Build history of the part. All positions in model axes, mm. A direction names the side the tool comes from. Coordinates: 2 decimals unless noted, no trailing zeros. Order: outer loops, then holes, each group sorted by start corner. A loop starts at its lowest first (then second) coordinate and runs counter-clockwise, first axis right, second up. Notation, with made-up numbers: (73.25, 74.25) - (129.25, 74.25) arc R25 cw to (129.25, 109.25) - close; hole circle Ø11 at (56.25, -35.75). An arc over 180 degrees is marked (long way). Return JSON: item names as keys, results as strings.
from build123d import *

# Parameters (mm, degrees)
SKETCH_1_W            = 62
SKETCH_1_H            = 98
EXTRUDE_1_DEPTH       = 8
CHAMFER_1_SIZE        = 1
HOLE_WIZARD_M4_1_D    = 4.8
CUT_EXTRUDE_1_DEPTH   = 3.3
MIRROR_2_COPY_1_D     = 4.8
MIRROR_2_COPY_2_DEPTH = 3.3


with BuildPart() as part:
    # ｽｹｯﾁ1 → ﾎﾞｽ - 押し出し1 (new body)
    with BuildSketch(Plane.XY):
        Rectangle(SKETCH_1_W, SKETCH_1_H)
    extrude(amount=EXTRUDE_1_DEPTH)

    # 面取り1
    chamfer_1_edges = [part.edges().sort_by_distance(p)[0] for p in [
        (0, -49, 0),
        (-31, 0, 0),
        (0, 49, 0),
        (31, 0, 0),
        (31, -49, 4),
        (-31, -49, 4),
        (-31, 49, 4),
        (31, 49, 4),
    ]]
    chamfer(chamfer_1_edges, length=CHAMFER_1_SIZE)

    # M4 すきま穴1 (through all)
    with Locations(Plane.XY.offset(8)):
        with Locations((-27.5, 44), (-27.5, 22), (-27.5, 0)):
            hole_wizard_m4_1 = Hole(HOLE_WIZARD_M4_1_D / 2)

    # ｽｹｯﾁ6 → ｶｯﾄ - 押し出し1 (cut)
    with BuildSketch(Plane(origin=(0, 0, 0), x_dir=(-1, 0, 0), z_dir=(0, 0, -1))):
        Polygon((27.5, 17.958548116), (31, 19.979274058), (31, 24.020725942), (27.5, 26.041451884), (24, 24.020725942), (24, 19.979274058), align=None)
        Polygon((27.5, 39.958548116), (31, 41.979274058), (31, 46.020725942), (27.5, 48.041451884), (24, 46.020725942), (24, 41.979274058), align=None)
        Polygon((27.5, -4.041451884), (31, -2.020725942), (31, 2.020725942), (27.5, 4.041451884), (24, 2.020725942), (24, -2.020725942), align=None)
    cut_extrude_1 = extrude(amount=-CUT_EXTRUDE_1_DEPTH, mode=Mode.SUBTRACT)

    # ﾐﾗｰ1: M4 すきま穴1, ｶｯﾄ - 押し出し1 across plane
    add(hole_wizard_m4_1.mirror(Plane.ZX), mode=Mode.SUBTRACT)
    add(cut_extrude_1.mirror(Plane.ZX), mode=Mode.SUBTRACT)

    # ﾐﾗｰ2: M4 すきま穴1, ｶｯﾄ - 押し出し1 across plane
    add(hole_wizard_m4_1.mirror(Plane(origin=(0, 0, 0), x_dir=(0, 0, 1), z_dir=(1, 0, 0))), mode=Mode.SUBTRACT)
    add(cut_extrude_1.mirror(Plane(origin=(0, 0, 0), x_dir=(0, 0, 1), z_dir=(1, 0, 0))), mode=Mode.SUBTRACT)

    # ﾐﾗｰ2 copy 1 (through all)
    with Locations(Plane(origin=(0, 0, 8), x_dir=(-1, 0, 0), z_dir=(0, 0, 1))):
        with Locations((-27.5, 44), (-27.5, 22), (-27.5, 0)):
            Hole(MIRROR_2_COPY_1_D / 2)

    # ﾐﾗｰ2 copy 2 sketch → ﾐﾗｰ2 copy 2 (cut)
    with BuildSketch(Plane(origin=(0, 0, 0), x_dir=(1, 0, 0), z_dir=(0, 0, -1))):
        Polygon((27.5, 17.958548116), (31, 19.979274058), (31, 24.020725942), (27.5, 26.041451884), (24, 24.020725942), (24, 19.979274058), align=None)
        Polygon((27.5, 39.958548116), (31, 41.979274058), (31, 46.020725942), (27.5, 48.041451884), (24, 46.020725942), (24, 41.979274058), align=None)
        Polygon((27.5, -4.041451884), (31, -2.020725942), (31, 2.020725942), (27.5, 4.041451884), (24, 2.020725942), (24, -2.020725942), align=None)
    extrude(amount=-MIRROR_2_COPY_2_DEPTH, mode=Mode.SUBTRACT)


solid = part.part
1. Cut at A-A on y = 0. Give the cut face in (x, z).
Check values:
{"outline": "(-31, 3.3) - (-29.9, 3.3) - (-29.9, 8) - (-31, 8) - close; (-25.1, 3.3) - (-24, 3.3) - (-24, 0) - (24, 0) - (24, 3.3) - (25.1, 3.3) - (25.1, 8) - (-25.1, 8) - close; (29.9, 3.3) - (31, 3.3) - (31, 8) - (29.9, 8) - close"}
2. Drop flat-ended pins along their axis: pin 1 (1.6 mm diameter, centred on y = -22, z = 1, fed in from -X); pin 2 (5.5 mm diameter, centred on x = -28, y = -0.5, fed in from -Z); pin 3 (3 mm diameter, centred on x = -27.5, y = 22, fed in from +Z). Give the stop position or say it passes through.
Check values:
{"pin 1": "x = -24", "pin 2": "z = 3.3", "pin 3": "through"}
3. Mould opens along X. For faces 5 (the flat face through (-24, 44, 2)), 6 (the cylindrical face through (-28.61, -19.87, 5.62)), 7 (the flat face through (31, -1, 5)) say: pulls with the +X half, pulls with the -X half, needs draft (parallel to the pull), parting line crosses it, or undercut.
Check values:
{"face 5": "pulls with the -X half", "face 6": "undercut", "face 7": "pulls with the +X half"}
4. Probe L1, parallel to Y at x = 27.5, z = 5.3; L2, parallel to Y at x = 26, z = 7.75. List the from-to ranges inside material, lowest first.
Check values:
{"L1": "-49 to -46.4, -41.6 to -24.4, -19.6 to -2.4, 2.4 to 19.6, 24.4 to 41.6, 46.4 to 49", "L2": "-49 to -45.87, -42.13 to -23.87, -20.13 to -1.87, 1.87 to 20.13, 23.87 to 42.13, 45.87 to 49"}
5. Cut at B-B on y = 23. Give the cut face in (x, z).
Check values:
{"outline": "(-31, 3.3) - (-29.68, 3.3) - (-29.68, 8) - (-31, 8) - close; (-25.32, 3.3) - (-24, 3.3) - (-24, 0) - (24, 0) - (24, 3.3) - (25.32, 3.3) - (25.32, 8) - (-25.32, 8) - close; (29.68, 3.3) - (31, 3.3) - (31, 8) - (29.68, 8) - close"}
6. Tool access for faces 1 (the flat face through (-24, 0, 2)), 2 (the cylindrical face through (28.61, -41.87, 5.62)), 3 (the flat face through (25.7, -3, 1.6)), 4 (the flat face through (24, 0, 2)): list every direction of +Z, -Z, +X, -X, +Y, -Y with a clear straight run to the whole face (end or side of a thin tool).
Check values:
{"face 1": "-Z, -X", "face 2": "+Z, -Z", "face 3": "-Z", "face 4": "-Z, +X"}
